Here's how the part is built. I have some questions about the finished solid (model axes, mm). A direction names the side the tool comes from. Coordinates: 2 decimals unless noted, no trailing zeros. Loops run counter-clockwise (first coordinate to the right, second up) from the corner with the lowest first, then second, coordinate; pieces in that order, holes last. Notation, with made-up numbers: M 56.25,-6.5 L 89.25,-6.5 A16 ccw 89.25,-2.5 Z; hole C -10,72 d6. An arc over 180 degrees is marked long. Use one line per item in the form item = value. Start each with the question number.
(1) Imagine slicing it at B-B, the plane y = 38. Please give me the cut outline in (x, z), and give its area (3 significant figures).
(2) On a 3-axis mill with a long thin cutter (end or side, diameter ignored), from which of +Z, -Z, +X, -X, +Y, -Y can I reach the whole of each face in a straight line? I mean faces 4 (the flat face through (0, 36, 10)), 5 (the cylindrical face through (0, 70, 5)), 6 (the flat face through (20, 33, 45)), 7 (the flat face through (-20, 32, 45)). Say none if no direction works.
(3) Please list where these lines run through material, in increasing order: L1, parallel to Z at x = -4, y = 17.5; L2, parallel to X at y = 34, z = 4.5; L3, parallel to Y at x = -33, z = 34.5.
(4) Thinking about a two-plate mould opening in Z: for faces 1 (the flat face through (20, 33, 5)), 2 (the flat face through (0, 36, 40)), 3 (the flat face through (1, 20, 50)), which applies, +Z half, -Z half, draft (parallel to the pull), parting line (faces both ways), or undercut?
(5) Will these pins go through, and if not, where does the flat tip stop? P1, Ø6, axis at x = -47.5, z = 26.5, coming from the +Y side; P2, Ø3, axis at y = 26, z = 3.5, coming from the +X side; P3, Ø3, axis at y = 30.5, z = 43, coming from the -X side.
(6) Imagine slicing it at A-A, the plane x = 0. Please give me the cut outline in (y, z), and give its area (3 significant figures).
(7) Imagine slicing it at C-C, the plane z = 31. Please give me the cut outline in (x, y), and give its area (3 significant figures).
(8) Imagine slicing it at D-D, the plane x = -48. Please give me the cut outline in (y, z).
```python
from build123d import *

# Parameters (mm, degrees)
BOSS_EXTRUDE1_DEPTH = 50
SKETCH2_R           = 10
CUT_EXTRUDE1_DEPTH  = 25
SKETCH2_3_R         = 10
CUT_EXTRUDE2_DEPTH  = 25
SKETCH3_W           = 40
SKETCH3_H           = 30
CUT_EXTRUDE3_DEPTH  = 99.742088291
SKETCH4_R           = 10
CUT_EXTRUDE4_DEPTH  = 108.819293264


with BuildPart() as part:
    # Sketch1 → Boss-Extrude1 (new body)
    with BuildSketch(Plane.XY):
        with BuildLine():
            Line((-65, 0), (-65, 15))
            Line((-65, 15), (-20, 15))
            Line((-20, 15), (-20, 50))
            ThreePointArc((-20, 50), (0, 70), (20, 50))
            Line((20, 50), (20, 15))
            Line((20, 15), (65, 15))
            Line((65, 15), (65, 0))
            Line((65, 0), (-65, 0))
        make_face()
    extrude(amount=BOSS_EXTRUDE1_DEPTH)

    # Sketch2 → Cut-Extrude1 (cut)
    with BuildSketch(Plane(origin=(0, 15, 0), x_dir=(1, 0, 0), z_dir=(0, 1, 0))):
        with Locations(Location((-40, -25, 0), (0, 0, 270))):
            Circle(SKETCH2_R)
    extrude(amount=-CUT_EXTRUDE1_DEPTH, mode=Mode.SUBTRACT)

    # Sketch2_3 → Cut-Extrude2 (cut)
    with BuildSketch(Plane(origin=(0, 15, 0), x_dir=(1, 0, 0), z_dir=(0, 1, 0))):
        with Locations(Location((40, -25, 0), (0, 0, 270))):
            Circle(SKETCH2_3_R)
    extrude(amount=-CUT_EXTRUDE2_DEPTH, mode=Mode.SUBTRACT)

    # Sketch3 → Cut-Extrude3 (cut, through all)
    with BuildSketch(Plane(origin=(0, 15, 0), x_dir=(1, 0, 0), z_dir=(0, 1, 0))):
        with Locations((0, -25)):
            Rectangle(SKETCH3_W, SKETCH3_H)
    extrude(amount=CUT_EXTRUDE3_DEPTH, mode=Mode.SUBTRACT)

    # Sketch4 → Cut-Extrude4 (cut, through all)
    with BuildSketch(Plane.XY.offset(50)):
        with Locations((0, 50)):
            Circle(SKETCH4_R)
    extrude(amount=-CUT_EXTRUDE4_DEPTH, mode=Mode.SUBTRACT)


solid = part.part
```
Answer:
q1.outline = M -20,0 L 20,0 L 20,10 L -20,10 Z; M -20,40 L 20,40 L 20,50 L -20,50 Z
q1.area = 800 mm²
q2.face_4 = +X, -X, +Y
q2.face_5 = +Z, -Z, +Y
q2.face_6 = +Z, -Z, +X, +Y
q2.face_7 = +Z, -Z, -X, +Y
q3.L1 = 0 to 10, 40 to 50
q3.L2 = -20 to 20
q3.L3 = 0 to 15
q4.face_1 = draft
q4.face_2 = undercut
q4.face_3 = +Z half
q5.P1 = 15
q5.P2 = 20
q5.P3 = -20
q6.outline = M 0,0 L 40,0 L 40,10 L 15,10 L 15,40 L 40,40 L 40,50 L 0,50 Z; M 60,0 L 70,0 L 70,10 L 60,10 Z; M 60,40 L 70,40 L 70,50 L 60,50 Z
q6.area = 1,450 mm²
q7.outline = M -65,0 L -48,0 L -48,15 L -65,15 Z; M -32,0 L 32,0 L 32,15 L -32,15 Z; M 48,0 L 65,0 L 65,15 L 48,15 Z
q7.area = 1,470 mm²
q8.outline = M 0,0 L 15,0 L 15,19 L 0,19 Z; M 0,31 L 15,31 L 15,50 L 0,50 Z
